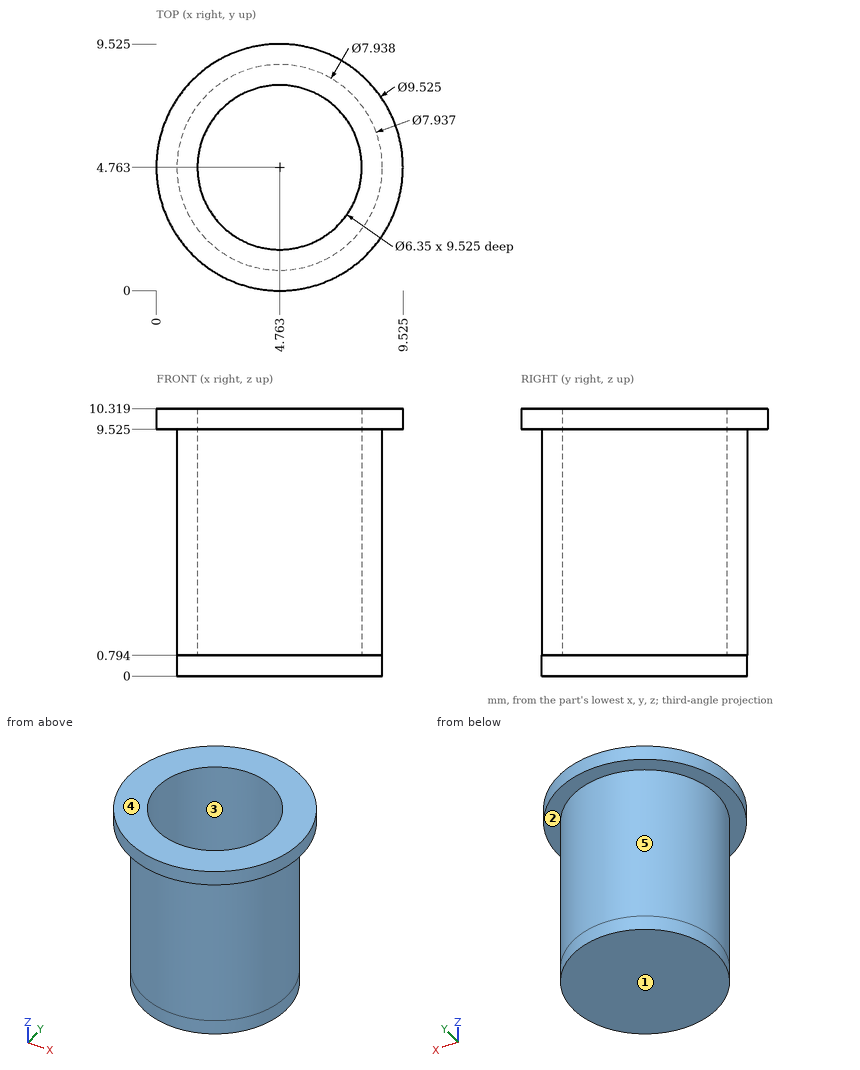
Check sheet for the drawn part. Datum: minimum x, y, z corner. Units: mm. A direction names the side the tool comes from. Round coordinates to 2 decimals unless told otherwise and drop trailing zeros. Use a Markdown table: item, result. Add a question column.
(1) Depth check by flat-ended pin: pin 1 (1 mm diameter, centred on y = 3, z = 1.5, fed in from -X); pin 2 (3 mm diameter, centred on x = 4, y = 5, fed in from +Z); pin 3 (5 mm diameter, centred on y = 8.5, z = 7, fed in from +X). Enter the tip coordinate at first touch or a pass-through.
(2) Material ranges on line 1 along Z through (x, y) = (2.25, 4); line 2 along Z through (x, y) = (7, 1) (1 decimal); line 3 along Y through (x, z) = (2.5, 3.5) (1 decimal), recorded low to high. Write a range as [from, to].
(3) Release check for a two-part mould opening along Y. For the marked faces 3, 4 and 5 record: pulls with the +Y half, pulls with the -Y half, needs draft (parallel to the pull), parting line crosses it, or undercut.
(4) Tool access check on the marked faces 1 and 2. Record the directions out of +Z, -Z, +X, -X, +Y, -Y that give a thin tool (end or side, any length) a straight path to the whole face; none if there is none.
Answers below:
| question | item | result |
|---|---|---|
| 1 | pin 1 | x = 1 |
| 1 | pin 2 | z = 0.79 |
| 1 | pin 3 | x = 8.53 |
| 2 | line 1 | [0, 0.79] |
| 2 | line 2 | [9.5, 10.3] |
| 2 | line 3 | [1.5, 2.5], [7, 8] |
| 3 | face 3 | undercut |
| 3 | face 4 | needs draft |
| 3 | face 5 | parting line crosses it |
| 4 | face 1 | -Z, +X, -X, +Y, -Y |
| 4 | face 2 | -Z |
